```python
from build123d import *

# Parameters (mm, degrees)
ESQUISSE1_R        = 15
ESQUISSE1_R_2      = 23.5
BOSS_EXTRU_1_DEPTH = 10
CONG_1_R           = 40


with BuildPart() as part:
    # Esquisse1 → Boss.-Extru.1 (new body)
    with BuildSketch(Plane.XY):
        Polygon((290, 0), (290, 55), (190, 120), (50, 120), (0, 78.045018441), (0, 0), (50, 0), (50, 10), (110, 10), (110, 0), (180, 0), (180, 10), (240, 10), (240, 0), align=None)
        with Locations((80, 80)):
            Circle(ESQUISSE1_R, mode=Mode.SUBTRACT)
        with Locations((216.747943312, 50)):
            Circle(ESQUISSE1_R_2, mode=Mode.SUBTRACT)
    extrude(amount=BOSS_EXTRU_1_DEPTH)

    # Congé1
    cong_1_edges = [part.edges().sort_by_distance(p)[0] for p in [
        (0, 78.045018441, 5),
        (50, 120, 5),
        (190, 120, 5),
        (290, 55, 5),
    ]]
    fillet(cong_1_edges, radius=CONG_1_R)


solid = part.part
```
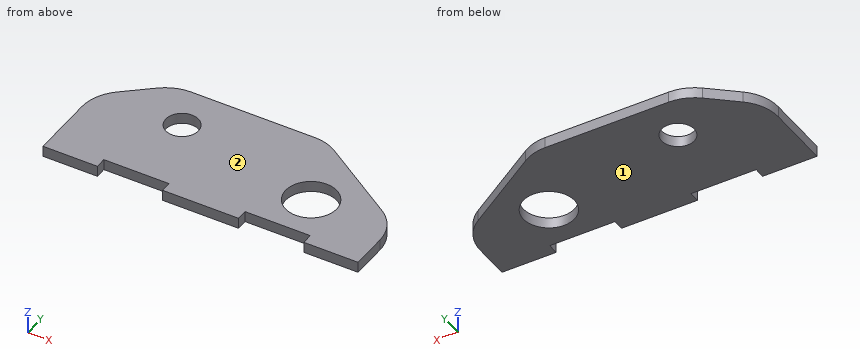
Could you check a few things on this model? Use its own coordinates, in mm. Face numbers are marked on the shaded views. Coordinates: 2 decimals unless noted, no trailing zeros. Write each loop counter-clockwise with the first axis right and the second up, starting at its lowest first coordinate (ties: lowest second). Pieces come first, ordered by that corner, then holes. Notation, with made-up numbers: M 62.5,-24 L 67.5,-24 A6 cw 67.5,-15 Z; hole C -36,82 d5. An arc over 180 degrees is marked long. Answer as CSV lines item,"result". Start each with the question number.
1) I want a section at A-A, the plane z = 5.25. Please give me the cut outline in (x, y).
2) For P1, Ø1.5, axis at y = 54.5, z = 8, coming from the +X side, with a flat end and sliding along its axis, tell me the tip position at first contact or that it passes through.
3) I want a section at D-D, the plane y = 104.5. Please give me the cut outline in (x, z), and give its area (3 significant figures).
4) Please list where these lines run through material, in increasing order: line 1 (Y direction, x = 80, z = 2.25); line 2 (Y direction, x = 103, z = 9); line 3 (Y direction, x = 87, z = 8.25). Write a range as from..to.
5) We'd pull the mould along Z, two halves only. Please class the marked faces 1 and 2: +Z half, -Z half, draft (parallel to the pull), parting line (faces both ways), or undercut.
6) I want a section at B-B, the plane x = 80. Please give me the cut outline in (y, z).
7) I want a section at C-C, the plane y = 80. Please give me the cut outline in (x, z).
Data:
1,outline,"M 0,0 L 50,0 L 50,10 L 110,10 L 110,0 L 180,0 L 180,10 L 240,10 L 240,0 L 290,0 L 290,33.29 A40 ccw 271.8,66.83 L 199.94,113.54 A40 ccw 178.14,120 L 64.56,120 A40 ccw 38.85,110.64 L 14.29,90.03 A40 ccw 0,59.39 Z; hole C 80,80 d30; hole C 216.75,50 d47"
2,P1,"stops at x = 284.37"
3,outline,"M 31.53,0 L 213.85,0 L 213.85,10 L 31.53,10 Z"
3,area,"1,820 mm^2"
4,line 1,"y = 10..65, 95..120"
4,line 2,"y = 10..120"
4,line 3,"y = 10..66.73, 93.27..120"
5,face 1,"-Z half"
5,face 2,"+Z half"
6,outline,"M 10,0 L 65,0 L 65,10 L 10,10 Z; M 95,0 L 120,0 L 120,10 L 95,10 Z"
7,outline,"M 5.72,0 L 65,0 L 65,10 L 5.72,10 Z; M 95,0 L 251.54,0 L 251.54,10 L 95,10 Z"
